```python
from build123d import *

# Parameters (mm, degrees)
CYLINDER150_R       = 1.7
CYLINDER150_DEPTH   = 11
CYLINDER154_R       = 7.14375
CYLINDER154_DEPTH   = 2.38125
CYLINDER155_R       = 9.525
CYLINDER155_DEPTH   = 2.38125
CYLINDER157_R       = 2.2
CYLINDER157_DEPTH   = 9
CYLINDER156_R       = 0.8
CYLINDER156_DEPTH   = 5
CYLINDER147_R       = 2.575
CYLINDER147_DEPTH   = 6
ARRAY_COUNT         = 3
CYLINDER151_R       = 1.7
CYLINDER151_DEPTH   = 11
BOX001_W            = 3
BOX001_H            = 6
BOX001_DEPTH        = 10.5
BOX_W               = 3
BOX_H               = 6
BOX_DEPTH           = 10.5
CYLINDER_R          = 3
CYLINDER_DEPTH      = 10.5
CYLINDER153_R       = 11
CYLINDER153_DEPTH   = 10.5
CYLINDER158_R       = 3
CYLINDER158_DEPTH   = 10.5
CUT_PLACEMENT_ANGLE = 180


with BuildPart() as obj1:
    # Cylinder150 → Cylinder150 (new body)
    with BuildSketch(Plane(origin=(-13, 0, 0), x_dir=(1, 0, 0), z_dir=(0, 0, 1))):
        Circle(CYLINDER150_R)
    extrude(amount=CYLINDER150_DEPTH)


with BuildPart() as cylinder008:
    # Cylinder154 → Cylinder154 (new body)
    with BuildSketch(Plane.XY):
        Circle(CYLINDER154_R)
    extrude(amount=CYLINDER154_DEPTH)


with BuildPart() as oring:
    # Cylinder155 → Cylinder155 (new body)
    with BuildSketch(Plane.XY):
        Circle(CYLINDER155_R)
    extrude(amount=CYLINDER155_DEPTH)

    # Cut019: cut Cylinder008
    add(cylinder008.part, mode=Mode.SUBTRACT)


with BuildPart() as oring_1:
    # Cut019 placement: moved
    add(oring.part.moved(Location((0, 0, -0.75))))


with BuildPart() as sealsubtraction:
    # Cylinder157 → Cylinder157 (new body)
    with BuildSketch(Plane.XY.offset(1.3)):
        Circle(CYLINDER157_R)
    extrude(amount=CYLINDER157_DEPTH)


with BuildPart() as bottomwireoutlet:
    # Cylinder156 → Cylinder156 (new body)
    with BuildSketch(Plane.XY.offset(-2)):
        Circle(CYLINDER156_R)
    extrude(amount=CYLINDER156_DEPTH)


with BuildPart() as sealarray:
    # Cylinder147 → Cylinder147 (new body)
    with BuildSketch(Plane.XY.offset(4.5)):
        Circle(CYLINDER147_R)
    extrude(amount=CYLINDER147_DEPTH)

    # Fusion: union SealSubtraction, BottomWireOutlet
    add(sealsubtraction.part)
    add(bottomwireoutlet.part)


with BuildPart() as sealarray_1:
    # Fusion placement: moved
    add(sealarray.part.moved(Location((4.25, 0, 0))))

    # Array: SealArray ×3 about axis
    array_axis = Axis((0, 0, 0), (0, 0, 1))


with BuildPart() as sealarray_2:
    add(sealarray_1.part)
    for i in range(1, ARRAY_COUNT):
        add(sealarray_1.part.rotate(array_axis, i * 360 / ARRAY_COUNT))


with BuildPart() as fusion002:
    # Cylinder151 → Cylinder151 (new body)
    with BuildSketch(Plane(origin=(13, 0, 0), x_dir=(1, 0, 0), z_dir=(0, 0, 1))):
        Circle(CYLINDER151_R)
    extrude(amount=CYLINDER151_DEPTH)

    # Fusion002: union obj1, Oring, SealArray
    add(obj1.part)
    add(oring_1.part)
    add(sealarray_2.part)


with BuildPart() as mountcube002:
    # Box001 → Box001 (new body)
    with BuildSketch(Plane(origin=(10, -3, 0), x_dir=(1, 0, 0), z_dir=(0, 0, 1))):
        with Locations((1.5, 3)):
            Rectangle(BOX001_W, BOX001_H)
    extrude(amount=BOX001_DEPTH)


with BuildPart() as mountcube1:
    # Box → Box (new body)
    with BuildSketch(Plane(origin=(-13, -3, 0), x_dir=(1, 0, 0), z_dir=(0, 0, 1))):
        with Locations((1.5, 3)):
            Rectangle(BOX_W, BOX_H)
    extrude(amount=BOX_DEPTH)


with BuildPart() as mountflange1:
    # Cylinder → Cylinder (new body)
    with BuildSketch(Plane(origin=(-13, 0, 0), x_dir=(1, 0, 0), z_dir=(0, 0, 1))):
        Circle(CYLINDER_R)
    extrude(amount=CYLINDER_DEPTH)


with BuildPart() as body:
    # Cylinder153 → Cylinder153 (new body)
    with BuildSketch(Plane.XY):
        Circle(CYLINDER153_R)
    extrude(amount=CYLINDER153_DEPTH)


with BuildPart() as cut:
    # Cylinder158 → Cylinder158 (new body)
    with BuildSketch(Plane(origin=(13, 0, 0), x_dir=(1, 0, 0), z_dir=(0, 0, 1))):
        Circle(CYLINDER158_R)
    extrude(amount=CYLINDER158_DEPTH)

    # Fusion001: union MountCube002, MountCube1, MountFlange1, Body
    add(mountcube002.part)
    add(mountcube1.part)
    add(mountflange1.part)
    add(body.part)

    # Cut: cut Fusion002
    add(fusion002.part, mode=Mode.SUBTRACT)


with BuildPart() as cut_1:
    # Cut placement: moved
    add(cut.part.rotate(Axis((0, 0, 0), (1, 0, 0)), CUT_PLACEMENT_ANGLE))


solid = cut_1.part
```
Geometry: final body of the model. Coordinates: model frame, mm. A direction names the side the tool comes from. Round coordinates to 2 decimals unless told otherwise and drop trailing zeros. Order: outer loops, then holes, each group sorted by start corner. A loop starts at its lowest first (then second) coordinate and runs counter-clockwise, first axis right, second up. Notation, with made-up numbers: M 29,18 L 77,18 A21 ccw 77,38 Z; hole C -32,8.25 d4. An arc over 180 degrees is marked long. Use one line per item in the form item = value. Start each with the question number.
Q1. Pin query (flat end, axial travel): pin 1 Ø5 at (x, z) = (3.5, -2) entering from +Y; pin 2 Ø1 at (y, z) = (-8, -3) entering from -X; pin 3 Ø1.2 at (x, z) = (-12, -7.5) entering from +Y. Return the tip coordinate at first contact, or that it passes through.
Q2. Cut plane A-A (y = 0). Count the separate pieces of the cut face and the enclosed holes in it, and give its area (3 significant figures).
Q3. Mould query, pull axis Y, two halves, no side actions, for faces 6 (the face through (-7.559, 5.796, -0.804)), 7 (the face through (3.45, -0.04, -0.64)), 8 (the face through (12, -3, -5)), 9 (the face through (12, 3, -5)). Classes: +Y half, -Y half, draft (parallel to the pull), parting line (faces both ways), or undercut.
Q4. Cut plane B-B (x = 4.25). Return loops of the section in (y, z) (3 decimals), and give its area (3 significant figures).
Q5. Access query for faces 1 (the face through (-12, 3, -5)), 2 (the face through (-7.137, -0.314, -0.804)), 3 (the face through (-2.3, -2.9, -0.6)), 4 (the face through (-1, -4, -1.3)), 5 (the face through (-12, -3, -5)). Directions: +Z, -Z, +X, -X, +Y, -Y. A direction counts if a zero-diameter tool reaches every point of the face in a straight line with its end or side. Return the directions, or none.
Q6. Cut plane D-D (y = -5). Return loops of the section in (x, z), and give its area (3 significant figures).
Q7. Material intervals for line 1 (X direction, y = 0, z = -7.85) (3 decimals); line 2 (X direction, y = 0, z = -3.25); line 3 (Y direction, x = -11.5, z = -2.5), sorted ascending. Write a range as [from, to].
Geometry results:
q1.pin_1 = 10.95
q1.pin_2 = -8.05
q1.pin_3 = 3
q2.separate_pieces = 4
q2.enclosed_holes = 0
q2.area = 210 mm^2
q3.face_6 = undercut
q3.face_7 = undercut
q3.face_8 = -Y half
q3.face_9 = +Y half
q4.outline = M -10.146,-10.5 L -2.575,-10.5 L -2.575,-4.5 L -2.2,-4.5 L -2.2,-1.3 L -0.8,-1.3 L -0.8,0 L -5.742,0 L -5.742,-1.631 L -8.524,-1.631 L -8.524,0 L -10.146,0 Z; M 0.8,-1.3 L 2.2,-1.3 L 2.2,-4.5 L 2.575,-4.5 L 2.575,-10.5 L 10.146,-10.5 L 10.146,0 L 8.524,0 L 8.524,-1.631 L 5.742,-1.631 L 5.742,0 L 0.8,0 Z
q4.area = 157 mm^2
q5.face_1 = +Z, -Z, -X, +Y
q5.face_2 = +Z
q5.face_3 = +Z, -Z
q5.face_4 = -Z
q5.face_5 = +Z, -Z, -X, -Y
q6.outline = M -9.8,-10.5 L -4.34,-10.5 L -4.34,-4.5 L -3.89,-4.5 L -3.89,-1.3 L -0.36,-1.3 L -0.36,-4.5 L 0.09,-4.5 L 0.09,-10.5 L 9.8,-10.5 L 9.8,0 L 8.11,0 L 8.11,-1.63 L 5.1,-1.63 L 5.1,0 L -5.1,0 L -5.1,-1.63 L -8.11,-1.63 L -8.11,0 L -9.8,0 Z
q6.area = 158 mm^2
q7.line_1 = [-16, -14.7], [-11.3, 1.675], [6.825, 11.3], [14.7, 16]
q7.line_2 = [-16, -14.7], [-11.3, 2.05], [6.45, 11.3], [14.7, 16]
q7.line_3 = [-3, -0.8], [0.8, 3]
